```python
from build123d import *

# Parameters (mm, degrees)
F0_R     = 5
F1_DEPTH = 25


with BuildPart() as f1:
    # F0 (on Top) → F1 (new body)
    with BuildSketch(Plane.XY):
        with BuildLine():
            Line((5.25788, 10.188084), (-9.74212, 10.188084))
            Line((-9.74212, 10.188084), (-9.74212, -9.811916))
            Line((-9.74212, -9.811916), (10.25788, -9.811916))
            Line((10.25788, -9.811916), (10.25788, 5.188084))
            ThreePointArc((10.25788, 5.188084), (8.793414, 8.723617), (5.25788, 10.188084))
        make_face()
        Circle(F0_R, mode=Mode.SUBTRACT)
    extrude(amount=F1_DEPTH)


solid = f1.part
```
Geometry: final body of the model. Coordinates: model frame, mm. Round coordinates to 2 decimals unless told otherwise and drop trailing zeros. Order: outer loops, then holes, each group sorted by start corner. A loop starts at its lowest first (then second) coordinate and runs counter-clockwise, first axis right, second up. Notation, with made-up numbers: (51, 35) - (89, 35) arc R14 ccw to (89, 55) - close; hole circle Ø5 at (60, -15.75). An arc over 180 degrees is marked (long way). Use CSV: the item, a comma, the result in double quotes. Start each with the question number.
Q1. Section query A-A (y = -3). Return loops of the section in (x, z).
Q2. Section query C-C (z = 23.75). Return loops of the section in (x, y), and give its area (3 significant figures).
Q3. Material intervals for line 1 along Y through (x, z) = (0, 11.5); line 2 along Y through (x, z) = (2, 7.25); line 3 along X through (y, z) = (3.75, 9.5), sorted ascending. Write a range as from..to.
Q4. Mould query, pull axis X, two halves, no side actions, for faces 1 (the face through (10.258, -2, 12)), 2 (the face through (-1.08, -4.88, 12.32)), 3 (the face through (-2, 10.188, 12)), 4 (the face through (-9.742, 0, 12)). Classes: +X half, -X half, draft (parallel to the pull), parting line (faces both ways), or undercut.
Q5. Section query B-B (x = 0). Return loops of the section in (y, z).
Q6. First-contact query: pin 1 (2 mm diameter, centred on x = -4.5, y = -6, fed in from -Z). Flat tip, straight axial feed; report the tip coordinate or a pass-through.
Q7. Section query D-D (x = 9.25). Return loops of the section in (y, z), and give its area (3 significant figures).
Result set:
1,outline,"(-9.74, 0) - (-4, 0) - (-4, 25) - (-9.74, 25) - close; (4, 0) - (10.26, 0) - (10.26, 25) - (4, 25) - close"
2,outline,"(-9.74, -9.81) - (10.26, -9.81) - (10.26, 5.19) arc R5 ccw to (5.26, 10.19) - (-9.74, 10.19) - close; hole circle Ø10 at (0, 0)"
2,area,"316 mm2"
3,line 1,"y = -9.81..-5, 5..10.19"
3,line 2,"y = -9.81..-4.58, 4.58..10.19"
3,line 3,"x = -9.74..-3.31, 3.31..10.26"
4,face 1,"+X half"
4,face 2,"undercut"
4,face 3,"draft"
4,face 4,"-X half"
5,outline,"(-9.81, 0) - (-5, 0) - (-5, 25) - (-9.81, 25) - close; (5, 0) - (10.19, 0) - (10.19, 25) - (5, 25) - close"
6,pin 1,"stops at z = 0"
7,outline,"(-9.81, 0) - (8.2, 0) - (8.2, 25) - (-9.81, 25) - close"
7,area,"450 mm2"
